Can you work these out from the model? Positions are in its coordinate system, mm. Face numbers are marked on the shaded views. Give positions to 0.01 mm unless a question says otherwise; leave off trailing zeros. Loops run counter-clockwise (first coordinate to the right, second up) from the corner with the lowest first, then second, coordinate; pieces in that order, holes last. Notation, with made-up numbers: (-32.75, 33.25) - (13.25, 33.25) arc R13 ccw to (13.25, 42.25) - close; hole circle Ø10 at (66, 67). An arc over 180 degrees is marked (long way). Use a Markdown table: item, result. Add a question column.
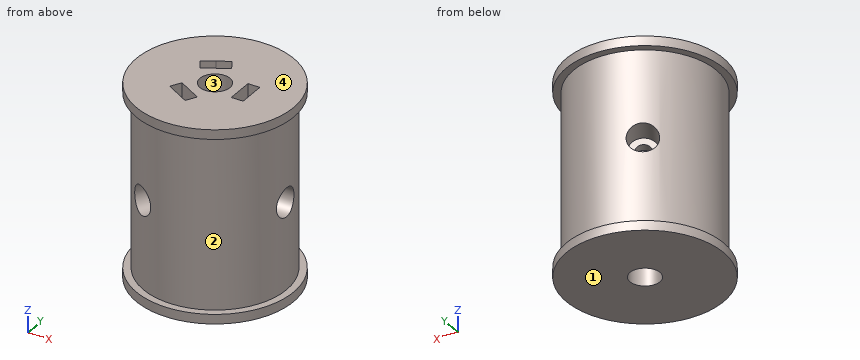
```python
from build123d import *

# Parameters (mm, degrees)
SKETCH1_R           = 15
SKETCH1_R_2         = 3.15
BOSS_EXTRUDE1_DEPTH = 40.3
CUT_EXTRUDE1_DEPTH  = 23
CUT_EXTRUDE4_REACH  = 37.49
SKETCH8_R           = 1.65
CUT_EXTRUDE5_REACH  = 37.49
SKETCH10_R          = 1.65
SKETCH12_R          = 3
CUT_EXTRUDE6_DEPTH  = 5.35
SKETCH15_R          = 3
CUT_EXTRUDE8_DEPTH  = 5.35
CUT_EXTRUDE9_REACH  = 37.49
SKETCH17_R          = 1.65
CUT_EXTRUDE10_REACH = 37.49
SKETCH18_R          = 1.65
SKETCH19_R          = 3
CUT_EXTRUDE11_DEPTH = 5.35
CUT_EXTRUDE12_REACH = 32
SKETCH20_R          = 1.65
CUT_EXTRUDE13_REACH = 32
SKETCH21_R          = 1.65
SKETCH22_R          = 16.5
SKETCH22_R_2        = 3.15
SKETCH22_W          = 2.5
SKETCH22_H          = 5.7
BOSS_EXTRUDE3_DEPTH = 2
SKETCH23_R          = 16.5
SKETCH23_R_2        = 3.15
BOSS_EXTRUDE4_DEPTH = 2


with BuildPart() as part:
    # Sketch1 → Boss-Extrude1 (new body)
    with BuildSketch(Plane.XY):
        Circle(SKETCH1_R)
        Circle(SKETCH1_R_2, mode=Mode.SUBTRACT)
    extrude(amount=BOSS_EXTRUDE1_DEPTH)

    # Sketch2 → Cut-Extrude1 (cut)
    with BuildSketch(Plane.XY.offset(40.3)):
        Polygon((7.65, 0), (7.65, 2.85), (5.15, 2.85), (5.15, -2.85), (7.65, -2.85), align=None)
        Polygon((-3.825, -6.625094339), (-1.356827599, -8.050094339), (-0.106827599, -5.885030829), (-5.043172401, -3.035030829), (-6.293172401, -5.200094339), align=None)
        Polygon((-3.825, 6.625094339), (-6.293172401, 5.200094339), (-5.048242412, 3.035349353), (-0.105426694, 5.882604512), (-1.356827546, 8.050094369), align=None)
    extrude(amount=-CUT_EXTRUDE1_DEPTH, mode=Mode.SUBTRACT)

    # Sketch8 → Cut-Extrude4 (cut, up to next)
    with BuildSketch(Plane(origin=(-7.5, -12.990381057, 0), x_dir=(0, 0, -1), z_dir=(-0.5, -0.866025404, 0)), mode=Mode.PRIVATE) as cut_extrude4_sk1:
        with Locations((-20.15, 0)):
            Circle(SKETCH8_R)
    cut_extrude4_tool1 = extrude(cut_extrude4_sk1.sketch, amount=-CUT_EXTRUDE4_REACH, mode=Mode.PRIVATE) & part.part
    add(cut_extrude4_tool1.solids().sort_by_distance((-7.5, -12.990381, 20.15))[0], mode=Mode.SUBTRACT)

    # Sketch10 → Cut-Extrude5 (cut, up to next)
    with BuildSketch(Plane(origin=(-7.5, -12.990381057, 0), x_dir=(0, 0, -1), z_dir=(-0.5, -0.866025404, 0)), mode=Mode.PRIVATE) as cut_extrude5_sk1:
        with Locations((-20.15, 0)):
            Circle(SKETCH10_R)
    cut_extrude5_tool1 = extrude(cut_extrude5_sk1.sketch, amount=-CUT_EXTRUDE5_REACH, mode=Mode.PRIVATE) & part.part
    add(cut_extrude5_tool1.solids().sort_by_distance((-7.5, -12.990381, 20.15))[0], mode=Mode.SUBTRACT)

    # Sketch12 → Cut-Extrude6 (cut)
    with BuildSketch(Plane(origin=(-7.5, -12.990381057, 0), x_dir=(0, 0, -1), z_dir=(-0.5, -0.866025404, 0))):
        with Locations((-20.15, 0)):
            Circle(SKETCH12_R)
    extrude(amount=-CUT_EXTRUDE6_DEPTH, mode=Mode.SUBTRACT)

    # Sketch15 → Cut-Extrude8 (cut)
    with BuildSketch(Plane(origin=(-7.5, 12.990381057, 0), x_dir=(0, 0, -1), z_dir=(-0.5, 0.866025404, 0))):
        with Locations((-20.15, 0)):
            Circle(SKETCH15_R)
    extrude(amount=-CUT_EXTRUDE8_DEPTH, mode=Mode.SUBTRACT)

    # Sketch17 → Cut-Extrude9 (cut, up to next)
    with BuildSketch(Plane(origin=(-7.5, 12.990381057, 0), x_dir=(0, 0, -1), z_dir=(-0.5, 0.866025404, 0)), mode=Mode.PRIVATE) as cut_extrude9_sk1:
        with Locations((-20.15, 0)):
            Circle(SKETCH17_R)
    cut_extrude9_tool1 = extrude(cut_extrude9_sk1.sketch, amount=-CUT_EXTRUDE9_REACH, mode=Mode.PRIVATE) & part.part
    add(cut_extrude9_tool1.solids().sort_by_distance((-7.5, 12.990381, 20.15))[0], mode=Mode.SUBTRACT)

    # Sketch18 → Cut-Extrude10 (cut, up to next)
    with BuildSketch(Plane(origin=(-7.5, 12.990381057, 0), x_dir=(0, 0, -1), z_dir=(-0.5, 0.866025404, 0)), mode=Mode.PRIVATE) as cut_extrude10_sk1:
        with Locations((-20.15, 0)):
            Circle(SKETCH18_R)
    cut_extrude10_tool1 = extrude(cut_extrude10_sk1.sketch, amount=-CUT_EXTRUDE10_REACH, mode=Mode.PRIVATE) & part.part
    add(cut_extrude10_tool1.solids().sort_by_distance((-7.5, 12.990381, 20.15))[0], mode=Mode.SUBTRACT)

    # Sketch19 → Cut-Extrude11 (cut)
    with BuildSketch(Plane(origin=(15, 0, 0), x_dir=(0, 0, -1), z_dir=(1, 0, 0))):
        with Locations((-20.15, 0)):
            Circle(SKETCH19_R)
    extrude(amount=-CUT_EXTRUDE11_DEPTH, mode=Mode.SUBTRACT)

    # Sketch20 → Cut-Extrude12 (cut, up to next)
    with BuildSketch(Plane(origin=(15, 0, 0), x_dir=(0, 0, -1), z_dir=(1, 0, 0)), mode=Mode.PRIVATE) as cut_extrude12_sk1:
        with Locations((-20.15, 0)):
            Circle(SKETCH20_R)
    cut_extrude12_tool1 = extrude(cut_extrude12_sk1.sketch, amount=-CUT_EXTRUDE12_REACH, mode=Mode.PRIVATE) & part.part
    add(cut_extrude12_tool1.solids().sort_by_distance((15, 0, 20.15))[0], mode=Mode.SUBTRACT)

    # Sketch21 → Cut-Extrude13 (cut, up to next)
    with BuildSketch(Plane(origin=(15, 0, 0), x_dir=(0, 0, -1), z_dir=(1, 0, 0)), mode=Mode.PRIVATE) as cut_extrude13_sk1:
        with Locations((-20.15, 0)):
            Circle(SKETCH21_R)
    cut_extrude13_tool1 = extrude(cut_extrude13_sk1.sketch, amount=-CUT_EXTRUDE13_REACH, mode=Mode.PRIVATE) & part.part
    add(cut_extrude13_tool1.solids().sort_by_distance((15, 0, 20.15))[0], mode=Mode.SUBTRACT)

    # Sketch22 → Boss-Extrude3 (add)
    with BuildSketch(Plane.XY.offset(40.3)):
        Circle(SKETCH22_R)
        Circle(SKETCH22_R_2, mode=Mode.SUBTRACT)
        Polygon((-1.356827599, -8.050094339), (-0.106827599, -5.885030829), (-5.043172401, -3.035030829), (-6.293172401, -5.200094339), align=None, mode=Mode.SUBTRACT)
        with Locations((6.4, 0)):
            Rectangle(SKETCH22_W, SKETCH22_H, mode=Mode.SUBTRACT)
        Polygon((-5.048242412, 3.035349353), (-0.105426694, 5.882604512), (-1.356827546, 8.050094369), (-6.293172401, 5.200094339), align=None, mode=Mode.SUBTRACT)
    extrude(amount=-BOSS_EXTRUDE3_DEPTH)

    # Sketch23 → Boss-Extrude4 (add)
    with BuildSketch(Plane(origin=(0, 0, 0), x_dir=(-1, 0, 0), z_dir=(0, 0, -1))):
        Circle(SKETCH23_R)
        Circle(SKETCH23_R_2, mode=Mode.SUBTRACT)
    extrude(amount=-BOSS_EXTRUDE4_DEPTH)


solid = part.part
```
1. Will these pins go through, and if not, where does the flat tip stop? P1, Ø3, axis at x = 5.5, z = 17, coming from the -Y side; P2, Ø6, axis at x = -3, z = 22, coming from the +Y side; P3, Ø8, axis at x = 9.5, z = 7.5, coming from the -Y side.
2. Suppose I cut it at B-B (z = 27). List the corners of the cut face in (x, y) for me (3 decimals), and give its area (3 significant figures).
3. If we mould it in two halves opening along Z, with no side actions, what happens to the marked faces 1, 2, 3 and 4? For each: released by +Z, released by -Z, zero draft, split by the parting line, or undercut.
4. Suppose I cut it at C-C (x = -13). List the corners of the cut face in (y, z) for me, and give its area (3 significant figures).
5. Please list where these lines run through material, in increasing order: line 1 along Z through (x, y) = (-10, -12); line 2 along Y through (x, z) = (0, 31); line 3 along Z through (x, y) = (4, -1.5). Write a range as [from, to].
6. Suppose I cut it at A-A (y = 0). State how many separate pieces and enclosed holes the cut face has, and give its area (3 significant figures).
Results below:
| question | item | result |
|---|---|---|
| 1 | P1 | y = -14.46 |
| 1 | P2 | y = 15 |
| 1 | P3 | y = -13.96 |
| 2 | outline | circle Ø30 at (0, 0); hole (-6.293, -5.2) - (-1.357, -8.05) - (-0.107, -5.885) - (-5.043, -3.035) - close; hole (-6.293, 5.2) - (-5.048, 3.035) - (-0.105, 5.883) - (-1.357, 8.05) - close; hole circle Ø6.3 at (0, 0); hole (5.15, -2.85) - (7.65, -2.85) - (7.65, 2.85) - (5.15, 2.85) - close |
| 2 | area | 633 mm² |
| 3 | face 1 | released by -Z |
| 3 | face 2 | undercut |
| 3 | face 3 | zero draft |
| 3 | face 4 | released by +Z |
| 4 | outline | (-10.16, 0) - (10.16, 0) - (10.16, 2) - (7.48, 2) - (7.48, 38.3) - (10.16, 38.3) - (10.16, 40.3) - (-10.16, 40.3) - (-10.16, 38.3) - (-7.48, 38.3) - (-7.48, 2) - (-10.16, 2) - close |
| 4 | area | 625 mm² |
| 5 | line 1 | [0, 2], [38.3, 40.3] |
| 5 | line 2 | [-15, -3.15], [3.15, 15] |
| 5 | line 3 | [0, 19.46], [20.84, 40.3] |
| 6 | separate pieces | 4 |
| 6 | enclosed holes | 0 |
| 6 | area | 864 mm² |
